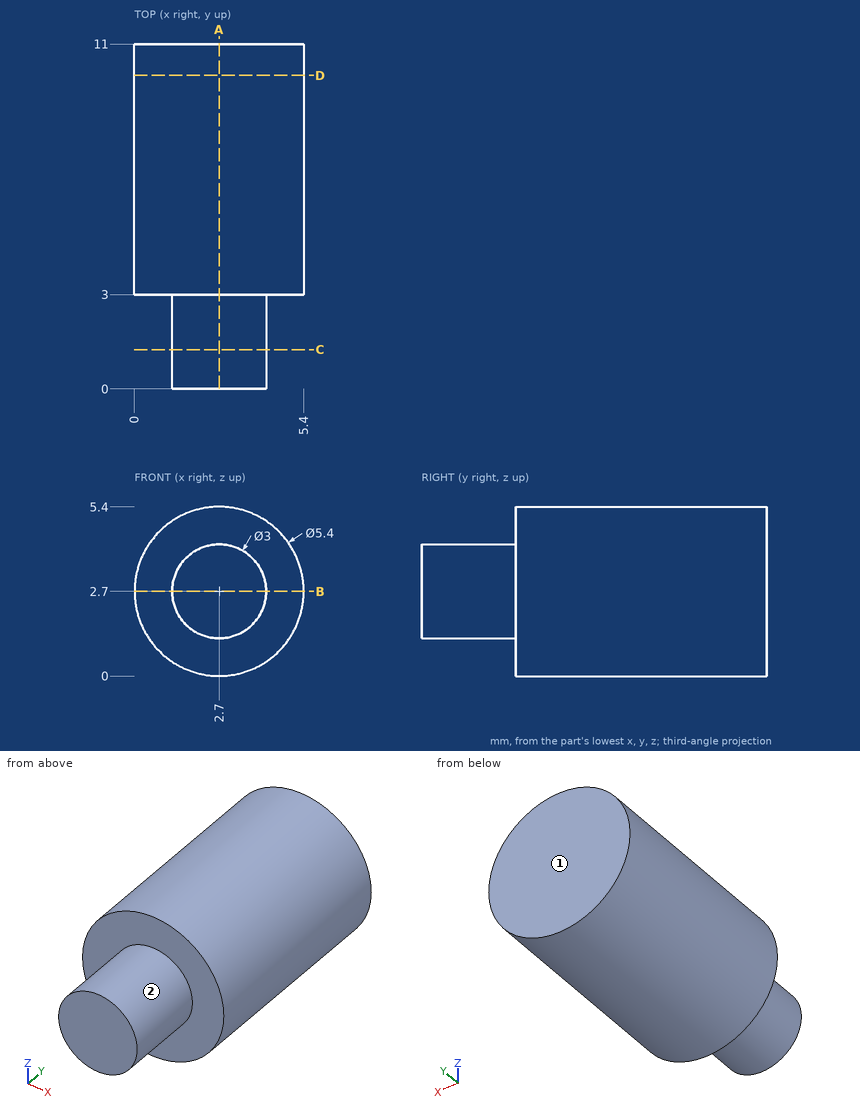
Could you check a few things on this drawing? It's one solid part, dimensions in mm from its lowest x, y, z. A direction names the side the tool comes from. Give positions to 0.01 mm unless a question says otherwise; leave off trailing zeros. Write each loop counter-clockwise with the first axis right and the second up, starting at its lowest first coordinate (ties: lowest second). Pieces come first, ordered by that corner, then holes. Notation, with made-up numbers: (32, -2) -> (55, -2) arc R22 ccw to (55, 26) -> close; hole circle Ø1 at (63.25, -13). An arc over 180 degrees is marked (long way). Answer as CSV lines item,"result". Start each with the question number.
(1) I'm going to push a flat-ended pin straight in: pin 1 Ø1 at (x, z) = (4.5, 1.5) entering from -Y. Where does the tip first touch, or does it pass through?
(2) If we section it at A-A, the plane x = 2.7: Write out the boundary of the cut face in (y, z), and give its area (3 significant figures).
(3) If we section it at B-B, the plane z = 2.7: Write out the boundary of the cut face in (x, y), and give its area (3 significant figures).
(4) Which directions (+Z, -Z, +X, -X, +Y, -Y) give clear straight access to the entire face, cutting with the end or side of a thin tool? Please do the marked faces 1 and 2.
(5) Please list where these lines run through material, in increasing order: line 1 (Z direction, x = 2.7, y = 1); line 2 (Y direction, x = 2.95, z = 4.3); line 3 (X direction, y = 2.5, z = 2.9).
(6) If we section it at D-D, the plane y = 10: Write out the boundary of the cut face in (x, z), and give its area (3 significant figures).
(7) If we section it at C-C, the plane y = 1.25: Write out the boundary of the cut face in (x, z), and give its area (3 significant figures).
Answer list:
1,pin 1,"y = 3"
2,outline,"(0, 1.2) -> (3, 1.2) -> (3, 0) -> (11, 0) -> (11, 5.4) -> (3, 5.4) -> (3, 4.2) -> (0, 4.2) -> close"
2,area,"52.2 mm^2"
3,outline,"(0, 3) -> (1.2, 3) -> (1.2, 0) -> (4.2, 0) -> (4.2, 3) -> (5.4, 3) -> (5.4, 11) -> (0, 11) -> close"
3,area,"52.2 mm^2"
4,face 1,"+Z, -Z, +X, -X, +Y"
4,face 2,"-Y"
5,line 1,"1.2 to 4.2"
5,line 2,"3 to 11"
5,line 3,"1.21 to 4.19"
6,outline,"circle Ø5.4 at (2.7, 2.7)"
6,area,"22.9 mm^2"
7,outline,"circle Ø3 at (2.7, 2.7)"
7,area,"7.07 mm^2"
